from build123d import *

# Parameters (mm, degrees)
F0_W     = 600
F0_H     = 2200
F0_W_2   = 520
F0_H_2   = 2120
F1_DEPTH = 600
F2_W     = 520
F2_H     = 520
F3_DEPTH = 40
F4_W     = 520
F4_H     = 2120
F5_DEPTH = 600


with BuildPart() as f1:
    # F0 (on Right) → F1 (new body)
    with BuildSketch(Plane.YZ):
        Rectangle(F0_W, F0_H)
        Rectangle(F0_W_2, F0_H_2, mode=Mode.SUBTRACT)
    extrude(amount=F1_DEPTH)

    # F2 (on face) → F3 (cut, through all)
    with BuildSketch(Plane.XY.offset(1100)):
        with Locations((300, 0)):
            Rectangle(F2_W, F2_H)
    extrude(amount=-F3_DEPTH, mode=Mode.SUBTRACT)

    # F4 (on face) → F5 (cut, through all)
    with BuildSketch(Plane(origin=(0, 300, 0), x_dir=(-1, 0, 0), z_dir=(0, 1, 0))):
        with Locations((-300, 0)):
            Rectangle(F4_W, F4_H)
    extrude(amount=-F5_DEPTH, mode=Mode.SUBTRACT)


solid = f1.part
Input: part model. Units: mm. Frame: model coordinates. A direction names the side the tool comes from. Give positions to 0.01 mm unless a question says otherwise; leave off trailing zeros. Loops run counter-clockwise (first coordinate to the right, second up) from the corner with the lowest first, then second, coordinate; pieces in that order, holes last. Notation, with made-up numbers: M 60.25,1.5 L 79.25,1.5 A7 ccw 79.25,5.5 Z; hole C -24,19 d3. An arc over 180 degrees is marked long. Use CSV: the item, a comma, the result in double quotes.
(1) Section C-C, the plane y = -118.5. Return loops of the section in (x, z).
Outcome:
outline,"M 0,-1100 L 600,-1100 L 600,-1060 L 0,-1060 Z; M 0,1060 L 40,1060 L 40,1100 L 0,1100 Z; M 560,1060 L 600,1060 L 600,1100 L 560,1100 Z"
(2) Pull-direction query (Y, two-part tool) for faces 1 (the face through (296, -4, -1100)), 2 (the face through (565, -300, -168)), 3 (the face through (296, -260, 1080)); classes: pulls with the +Y half, pulls with the -Y half, needs draft (parallel to the pull), parting line crosses it, or undercut.
Outcome:
face 1,"needs draft"
face 2,"pulls with the -Y half"
face 3,"undercut"
(3) Material intervals for L1, parallel to X at y = 268.5, z = -130; L2, parallel to Z at x = 465.5, y = 47.5; L3, parallel to Y at x = 26, z = 556.5, sorted ascending. Write a range as [from, to].
Outcome:
L1,"x = [0, 40], [560, 600]"
L2,"z = [-1100, -1060]"
L3,"y = [-300, -260], [260, 300]"
(4) Section A-A, the plane z = 702.5. Return loops of the section in (x, y), plus the area to 3 significant figures.
Outcome:
outline,"M 0,-300 L 40,-300 L 40,-260 L 0,-260 Z; M 0,260 L 40,260 L 40,300 L 0,300 Z; M 560,-300 L 600,-300 L 600,-260 L 560,-260 Z; M 560,260 L 600,260 L 600,300 L 560,300 Z"
area,"6,400 mm²"
(5) Pin query (flat end, axial travel): P1, Ø1, axis at x = 320, y = 173.5, coming from the +Z side. Return the tip coordinate at first contact, or that it passes through.
Outcome:
P1,"stops at z = -1060"
(6) Set-up query: faces 4 (the face through (560, 280, -15)), 5 (the face through (562, -4, 1100)), 6 (the face through (296, 260, 1080)), 7 (the face through (580, -260, 15)), 8 (the face through (600, -268, 168)). Return all of +Z, -Z, +X, -X, +Y, -Y with unobstructed straight access to the full face (end or side cutting, diameter ignored); none if empty.
Outcome:
face 4,"+Y, -Y"
face 5,"+Z, +X, -X, +Y, -Y"
face 6,"+Z"
face 7,"+X, -X"
face 8,"+Z, -Z, +X, +Y, -Y"
(7) Section B-B, the plane x = 455. Return loops of the section in (y, z), plus the area to 3 significant figures.
Outcome:
outline,"M -300,-1100 L 300,-1100 L 300,-1060 L -300,-1060 Z; M -300,1060 L -260,1060 L -260,1100 L -300,1100 Z; M 260,1060 L 300,1060 L 300,1100 L 260,1100 Z"
area,"27,200 mm²"
